from build123d import *

# Parameters (mm, degrees)
F1_DEPTH = 812.8
F2_W     = 76.2
F2_H     = 431.8
F3_DEPTH = 76.2
F4_W     = 549.230704
F4_H     = 403.036444
F5_DEPTH = 127
F6_R     = 38.1
F7_DEPTH = 25.4
F8_R     = 22.936038
F9_DEPTH = 50.8


with BuildPart() as f1:
    # F0 (on Front) → F1 (new body)
    with BuildSketch(Plane.XZ):
        Polygon((327.509973, 1525.438145), (327.509973, 1741.338145), (-156.425023, 1461.938145), (-156.425023, -277.961855), (681.774977, -277.961855), (681.774977, 522.138145), (516.674977, 522.138145), (516.674977, 712.638145), (176.990611, 1187.931919), (176.990611, 1391.131919), align=None)
    extrude(amount=-F1_DEPTH)

    # F2 (on face) → F3 (cut)
    with BuildSketch(Plane(origin=(-612.619926, 0, 686.57398), x_dir=(0.74615, 0, 0.665778), z_dir=(0.665778, 0, -0.74615))):
        with Locations((1176.240321, -406.003956)):
            Rectangle(F2_W, F2_H)
    extrude(amount=-F3_DEPTH, mode=Mode.SUBTRACT)

    # F4 (on face) → F5 (cut)
    with BuildSketch(Plane(origin=(679.11339, 0, 485.350775), x_dir=(0, 1, 0), z_dir=(0.813581, 0, 0.581452))):
        with Locations((406.4, 571.46676)):
            Rectangle(F4_W, F4_H)
    extrude(amount=-F5_DEPTH, mode=Mode.SUBTRACT)

    # F6 (on face) → F7 (cut)
    with BuildSketch(Plane.YZ.offset(176.990611)):
        with Locations((406.4, 1281.323433)):
            Circle(F6_R)
    extrude(amount=-F7_DEPTH, mode=Mode.SUBTRACT)

    # F8 (on face) → F9 (cut)
    with BuildSketch(Plane.YZ.offset(516.674977)):
        with Locations((406.476498, 552.552164)):
            Circle(F8_R)
    extrude(amount=-F9_DEPTH, mode=Mode.SUBTRACT)


solid = f1.part
For this review, take the finished solid that the model builds, in its own axes (mm). A direction names the side the tool comes from. Round coordinates to 2 decimals unless told otherwise and drop trailing zeros. Loops run counter-clockwise (first coordinate to the right, second up) from the corner with the lowest first, then second, coordinate; pieces in that order, holes last. Notation, with made-up numbers: (-36.5, -27) - (18.5, -27) arc R24 ccw to (18.5, 11) - close; hole circle Ø9 at (-17.5, 68.5). An arc over 180 degrees is marked (long way). Use one line per item in the form item = value.
1) Wall thickness on probe 1 along Z at (x, y) = (160.25, 406.4); probe 2 along Z at (x, y) = (258, 59.5); probe 3 along Z at (x, y) = (268.5, 279.5): over which ranges is each line inside the solid? List them lowest first.
Solutions:
probe_1 = -277.96 to 992.94, 1064.63 to 1243.22, 1319.42 to 1644.77
probe_2 = -277.96 to 1074.58, 1463.42 to 1701.21
probe_3 = -277.96 to 841.47, 1523.03 to 1707.27
2) Tool access review of faces 4 (the face through (600, 401, 522.138)), 5 (the face through (234, 401, 1442)), 6 (the face through (298, 681.015, 912)), 7 (the face through (491.631, 388.275, 538.596)), 8 (the face through (413.07, 402.56, 749.93)): name each direction out of +Z, -Z, +X, -X, +Y, -Y from which nothing blocks a thin tool from reaching the whole face with its end or side.
Solutions:
face_4 = +Z, +X, +Y, -Y
face_5 = +X, +Y, -Y
face_6 = none
face_7 = +X
face_8 = +Z
3) Mouldability with a two-part tool opening along Y and no side actions: class faces 1 (the face through (349.21, 129.78, 946.96)), 2 (the face through (164, 812.8, 521)), 3 (the face through (164.47, 398.14, 1244.13)) as pulls with the +Y half, pulls with the -Y half, needs draft (parallel to the pull), parting line crosses it, or undercut.
Solutions:
face_1 = needs draft
face_2 = pulls with the +Y half
face_3 = undercut
4) We need section B-B on z = 979. Write out the cut boundary in (x, y), then the cut area to 3 significant figures.
Solutions:
outline = (-156.43, 0) - (326.31, 0) - (326.31, 131.78) - (170.21, 131.78) - (170.21, 681.02) - (326.31, 681.02) - (326.31, 812.8) - (-156.43, 812.8) - close
area = 307,000 mm2
5) Clearance check with flat-ended pins moving along their axes: P1, Ø6, axis at y = 255, z = 1182, coming from the +X side; P2, Ø4, axis at x = -41, y = 560, coming from the +Z side; P3, Ø12, axis at x = 232.5, y = 313.5, coming from the +Z side. State where each tip first meets the part, or that it passes through.
Solutions:
P1 = 183.37
P2 = 1529.73
P3 = 1689.95
6) We need section C-C on y = 734.5. Write out the cut boundary in (x, z).
Solutions:
outline = (-156.43, -277.96) - (681.77, -277.96) - (681.77, 522.14) - (516.67, 522.14) - (516.67, 712.64) - (176.99, 1187.93) - (176.99, 1391.13) - (327.51, 1525.44) - (327.51, 1741.34) - (-156.43, 1461.94) - close
7) We need section D-D on x = -83. Write out the cut boundary in (y, z).
Solutions:
outline = (0, -277.96) - (812.8, -277.96) - (812.8, 1504.33) - (0, 1504.33) - close
8) We need section A-A on y = 252. Write out the cut boundary in (x, z).
Solutions:
outline = (-156.43, -277.96) - (681.77, -277.96) - (681.77, 522.14) - (516.67, 522.14) - (516.67, 712.64) - (464.01, 786.33) - (360.68, 712.49) - (126.34, 1040.39) - (229.66, 1114.24) - (176.99, 1187.93) - (176.99, 1391.13) - (236.6, 1444.32) - (185.87, 1501.18) - (242.73, 1551.91) - (293.46, 1495.06) - (327.51, 1525.44) - (327.51, 1741.34) - (-156.43, 1461.94) - close
